Could you check a few things on this model? Use its own coordinates, in mm. Face numbers are marked on the shaded views. A direction names the side the tool comes from. Coordinates: 2 decimals unless noted, no trailing zeros. Write each loop counter-clockwise with the first axis right and the second up, starting at its lowest first coordinate (ties: lowest second). Pieces come first, ordered by that corner, then holes.
Item 1: I want a section at C-C on z = -1.25. Please give me the cut outline in (x, y), then the cut area to 3 significant figures.
Item 2: I want a section at B-B on y = 46.5. Please give me the cut outline in (x, z), then the cut area to 3 significant figures.
Item 3: Which directions (+Z, -Z, +X, -X, +Y, -Y) give clear straight access to the entire face, cutting with the end or side of a thin tool? Please do the marked faces 4 and 5.
Item 4: I want a section at A-A on x = 49. Please give me the cut outline in (y, z), then the cut area to 4 significant figures.
Item 5: For P1, Ø2.5, axis at x = 73.5, z = -4, coming from the +Y side; P2, Ø0.6, axis at y = 64.5, z = -5, coming from the +X side; P3, Ø4, axis at y = 14.5, z = -8, coming from the +X side, each with a flat end and sliding along its axis, tell me the tip position at first contact or that it passes through.
Item 6: If I drill on probe 1 along Y at (x, z) = (40.5, -2.5); probe 2 along Y at (x, z) = (49.5, -5.5); probe 3 along Y at (x, z) = (8.5, -1.5), over which ranges is the centre line in solid material (lowest first)?
Item 7: I want a section at D-D on x = 41. Please give me the cut outline in (y, z).
Item 8: Thinking about a two-plate mould opening in Y: for the marked faces 1, 2 and 3, which applies, +Y half, -Y half, draft (parallel to the pull), parting line (faces both ways), or undercut?
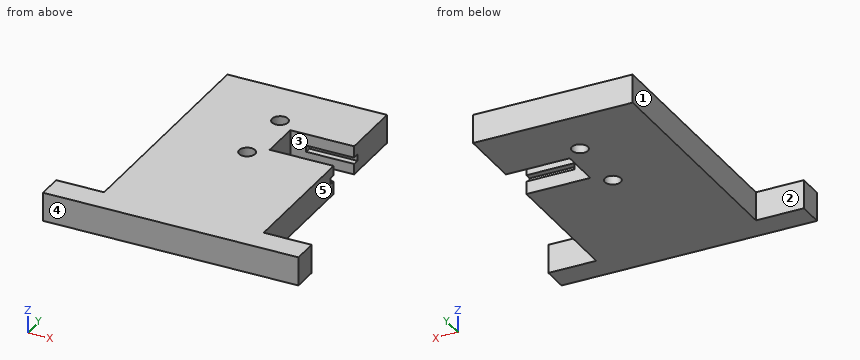
from build123d import *

# Parameters (mm, degrees)
ESQUISSE1_R             = 2.5
BOSS_EXTRU_1_DEPTH      = 9
ESQUISSE2_W             = 9
ESQUISSE2_H             = 12.5
ENL_V_MAT_EXTRU_2_DEPTH = 20
ESQUISSE4_W             = 15
ESQUISSE4_H             = 2
ENL_V_MAT_EXTRU_4_DEPTH = 2
ESQUISSE6_W             = 15
ESQUISSE6_H             = 2
ENL_V_MAT_EXTRU_5_DEPTH = 2


with BuildPart() as part:
    # Esquisse1 → Boss.-Extru.1 (new body)
    with BuildSketch(Plane.XY):
        Polygon((1.553236782, 0), (81.553236782, 0), (81.553236782, 8), (66.553236782, 8), (66.553236782, 83), (16.553236782, 83), (16.553236782, 8), (1.553236782, 8), align=None)
        with Locations((41.553236782, 46.5)):
            Circle(ESQUISSE1_R, mode=Mode.SUBTRACT)
        with Locations((41.553236782, 66.5)):
            Circle(ESQUISSE1_R, mode=Mode.SUBTRACT)
    extrude(amount=-BOSS_EXTRU_1_DEPTH)

    # Esquisse2 → Enlèv. mat.-Extru.2 (cut)
    with BuildSketch(Plane(origin=(66.553236782, 0, 0), x_dir=(0, 0, -1), z_dir=(1, 0, 0))):
        with Locations((4.5, 56.75)):
            Rectangle(ESQUISSE2_W, ESQUISSE2_H)
    extrude(amount=-ENL_V_MAT_EXTRU_2_DEPTH, mode=Mode.SUBTRACT)

    # Esquisse4 → Enlèv. mat.-Extru.4 (cut)
    with BuildSketch(Plane(origin=(0, 50.5, 0), x_dir=(1, 0, 0), z_dir=(0, 1, 0))):
        with Locations((59.053236782, 3.973765147)):
            Rectangle(ESQUISSE4_W, ESQUISSE4_H)
    extrude(amount=-ENL_V_MAT_EXTRU_4_DEPTH, mode=Mode.SUBTRACT)

    # Esquisse6 → Enlèv. mat.-Extru.5 (cut)
    with BuildSketch(Plane.XZ.offset(-63)):
        with Locations((59.053236782, -4.638650815)):
            Rectangle(ESQUISSE6_W, ESQUISSE6_H)
    extrude(amount=-ENL_V_MAT_EXTRU_5_DEPTH, mode=Mode.SUBTRACT)


solid = part.part
Response values:
1. outline: (1.55, 0) - (81.55, 0) - (81.55, 8) - (66.55, 8) - (66.55, 50.5) - (46.55, 50.5) - (46.55, 63) - (66.55, 63) - (66.55, 83) - (16.55, 83) - (16.55, 8) - (1.55, 8) - close; hole circle Ø5 at (41.55, 46.5); hole circle Ø5 at (41.55, 66.5)
1. area: 4,100 mm2
2. outline: (16.55, -9) - (39.05, -9) - (39.05, 0) - (16.55, 0) - close; (44.05, -9) - (66.55, -9) - (66.55, 0) - (44.05, 0) - close
2. area: 405 mm2
3. face 4: +Z, -Z, +X, -X, -Y
3. face 5: +Z, -Z, +X, +Y
4. outline: (0, -9) - (50.5, -9) - (50.5, 0) - (0, 0) - close; (63, -9) - (83, -9) - (83, 0) - (63, 0) - close
4. area: 634.5 mm2
5. P1: stops at y = 8
5. P2: stops at x = 51.55
5. P3: stops at x = 66.55
6. probe 1: y = 0 to 44.23, 48.77 to 64.23, 68.77 to 83
6. probe 2: y = 0 to 50.5, 63 to 83
6. probe 3: y = 0 to 8
7. outline: (0, -9) - (44.06, -9) - (44.06, 0) - (0, 0) - close; (48.94, -9) - (64.06, -9) - (64.06, 0) - (48.94, 0) - close; (68.94, -9) - (83, -9) - (83, 0) - (68.94, 0) - close
8. face 1: draft
8. face 2: +Y half
8. face 3: undercut
